Geometry check sheet. Reference: the model listing, model coordinates, mm. Face numbers are marked on the shaded views. A direction names the side the tool comes from. Round coordinates to 2 decimals unless told otherwise and drop trailing zeros. Write each loop counter-clockwise with the first axis right and the second up, starting at its lowest first coordinate (ties: lowest second). Pieces come first, ordered by that corner, then holes. Notation, with made-up numbers: M 67,-26.5 L 71,-26.5 A20 ccw 71,11.5 Z; hole C 2.25,72 d2. An arc over 180 degrees is marked long. Put each result on its own line as item: value. Start each with the question number.
(1) Tool access check on the marked faces 1 and 2. Record the directions out of +Z, -Z, +X, -X, +Y, -Y that give a thin tool (end or side, any length) a straight path to the whole face; none if there is none.
(2) Section check B-B on y = 19. Record the cut outline in (x, z), then the cut area to 3 significant figures.
(3) Mould release check, pull along X, two halves, no side actions. Record for the marked faces 3, 4, 5 and 6: pulls with the +X half, pulls with the -X half, needs draft (parallel to the pull), parting line crosses it, or undercut.
(4) Section check D-D on z = -12. Record the cut outline in (x, y) (1 decimal), then the cut area to 3 significant figures.
(5) Section check C-C on z = -29. Record the cut outline in (x, y) (1 decimal), then the cut area to 3 significant figures.
(6) Gauge pin test, flat end, axial feed: pin 1 (1.9 mm diameter, centred on x = -54.5, y = -25.5, fed in from +Z). Record the tip position at first contact, or that the pin passes through.
(7) Material ranges on probe 1 along Y at (x, z) = (-43.5, -3) (3 decimals); probe 2 along X at (y, z) = (40.5, -17); probe 3 along X at (y, z) = (54.5, -34), recorded low to high.
(8) Section check A-A on x = -46.5. Record the cut outline in (y, z) (3 decimals).
from build123d import *

# Parameters (mm, degrees)
SKETCH2_W           = 136.525
SKETCH2_H           = 127
BOSS_EXTRUDE1_DEPTH = 38.1
SKETCH3_W           = 117.475
SKETCH3_H           = 120.65
CUT_EXTRUDE2_DEPTH  = 31.75
SKETCH4_W           = 104.775
SKETCH4_H           = 120.65
CUT_EXTRUDE3_DEPTH  = 38.1
SKETCH5_R           = 2.8448
CUT_EXTRUDE4_DEPTH  = 25.4


with BuildPart() as part:
    # Sketch2 → Boss-Extrude1 (new body)
    with BuildSketch(Plane.XY):
        Rectangle(SKETCH2_W, SKETCH2_H)
    extrude(amount=-BOSS_EXTRUDE1_DEPTH)

    # Sketch3 → Cut-Extrude2 (cut)
    with BuildSketch(Plane.XY):
        Rectangle(SKETCH3_W, SKETCH3_H)
    extrude(amount=-CUT_EXTRUDE2_DEPTH, mode=Mode.SUBTRACT)

    # Sketch4 → Cut-Extrude3 (cut)
    with BuildSketch(Plane(origin=(0, 0, -38.1), x_dir=(-1, 0, 0), z_dir=(0, 0, -1))):
        Rectangle(SKETCH4_W, SKETCH4_H)
    extrude(amount=-CUT_EXTRUDE3_DEPTH, mode=Mode.SUBTRACT)

    # Sketch5 → Cut-Extrude4 (cut)
    with BuildSketch(Plane.XY):
        with Locations((-63.62065, 59.182)):
            Circle(SKETCH5_R)
        with Locations(Location((63.62065, 59.182, 0), (0, 0, 180))):
            Circle(SKETCH5_R)
        with Locations((63.62065, -59.182)):
            Circle(SKETCH5_R)
        with Locations(Location((-63.62065, -59.182, 0), (0, 0, 180))):
            Circle(SKETCH5_R)
    extrude(amount=-CUT_EXTRUDE4_DEPTH, mode=Mode.SUBTRACT)


solid = part.part
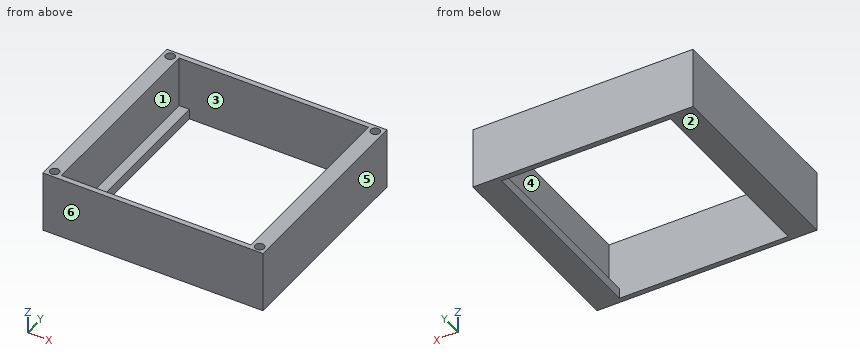
Answers follow:
1. face 1: +Z
1. face 2: -Z, +X, -X, +Y, -Y
2. outline: M -68.26,-38.1 L -52.39,-38.1 L -52.39,-31.75 L -58.74,-31.75 L -58.74,0 L -68.26,0 Z; M 52.39,-38.1 L 68.26,-38.1 L 68.26,0 L 58.74,0 L 58.74,-31.75 L 52.39,-31.75 Z
2. area: 806 mm^2
3. face 3: undercut
3. face 4: undercut
3. face 5: pulls with the +X half
3. face 6: needs draft
4. outline: M -68.3,-63.5 L 68.3,-63.5 L 68.3,63.5 L -68.3,63.5 Z; hole C -63.6,-59.2 d5.7; hole C -63.6,59.2 d5.7; hole M -58.7,-60.3 L 58.7,-60.3 L 58.7,60.3 L -58.7,60.3 Z; hole C 63.6,-59.2 d5.7; hole C 63.6,59.2 d5.7
4. area: 3,060 mm^2
5. outline: M -68.3,-63.5 L 68.3,-63.5 L 68.3,63.5 L -68.3,63.5 Z; hole M -58.7,-60.3 L 58.7,-60.3 L 58.7,60.3 L -58.7,60.3 Z
5. area: 3,170 mm^2
6. pin 1: stops at z = -31.75
7. probe 1: y = -63.5 to -60.325, 60.325 to 63.5
7. probe 2: x = -68.26 to -58.74, 58.74 to 68.26
7. probe 3: x = -68.26 to -52.39, 52.39 to 68.26
8. outline: M -63.5,-38.1 L -60.325,-38.1 L -60.325,0 L -63.5,0 Z; M 60.325,-38.1 L 63.5,-38.1 L 63.5,0 L 60.325,0 Z
